Autodesk Inventor part; units mm, degrees
ref_plane "YZ Plane" through (0, 0, 0) normal (1, 0, 0) x (0, 1, 0)
ref_plane "XZ Plane" through (0, 0, 0) normal (0, 1, 0) x (-1, 0, 0)
ref_plane "XY Plane" through (0, 0, 0) normal (0, 0, 1) x (1, 0, 0)
sketch "Sketch1" plane through (0, 0, 0) normal (1, 0, 0) x (0, 1, 0)
  line L0 (0, 0) -> (0, -3.5)
  line L1 (0, -3.5) -> (1.3, -3.5)
  line L2 (1.3, -3.5) -> (1.3, -3.25)
  line L3 (1.3, -3.25) -> (2.3425, -3.25)
  line L4 (2.3425, -3.25) -> (2.3425, -3.5)
  line L5 (2.3425, -3.5) -> (3.6425, -3.5)
  line L6 (3.6425, -3.5) -> (3.6425, -3.25)
  line L7 (3.6425, -3.25) -> (5, -3.25)
  line L8 (5, -3.25) -> (5, 0)
  line L9 (5, 0) -> (0, 0)
  line L10 (5, -2.5) -> (0, -2.5)
  point P0 (1.8212, -3.25)
  dimension "d0" = 3.25
  dimension "d1" = 5
  dimension "d2" = 3.5
  dimension "d3" = 1.3
  dimension "d4" = 1.3
  dimension "d5" = 2.5
revolve "Revolution1" add sketch "Sketch1" angle 360 about axis through (0, 5, 0) along (0, -1, 0) contours L10 L8 L7 L6 L5 L4 L3 L2 L1 L0
equation "\"d4\" = d3"
properties part number "M5 heat set inserts"
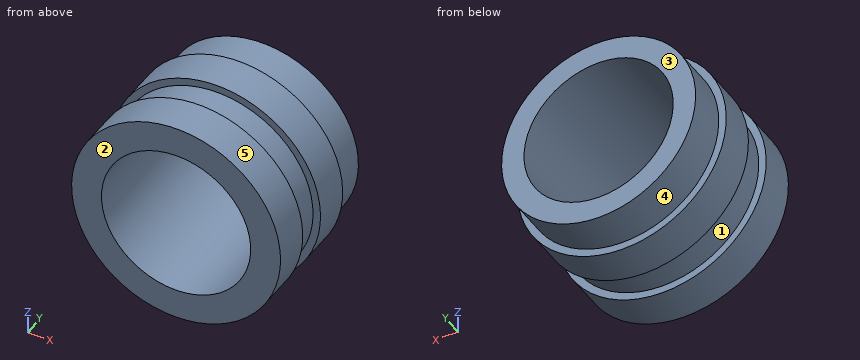
Check sheet for the modelled part. Datum: model origin and axes. Units: mm. Face numbers are marked on the shaded views. A direction names the side the tool comes from. Round coordinates to 2 decimals unless told otherwise and drop trailing zeros. Order: outer loops, then holes, each group sorted by start corner. A loop starts at its lowest first (then second) coordinate and runs counter-clockwise, first axis right, second up.
Q1. Draft check along Y on the marked faces 1, 2 and 3. Enter one of: pulls with the +Y half, pulls with the -Y half, needs draft (parallel to the pull), parting line crosses it, or undercut.
Filled sheet:
face 1: undercut
face 2: pulls with the -Y half
face 3: pulls with the +Y half
Q2. Cross-section at B-B, the plane z = 0. Enter the section's corners in (x, y), plus the area to 3 significant figures.
Filled sheet:
outline: (-3.5, 0) - (-2.5, 0) - (-2.5, 5) - (-3.25, 5) - (-3.25, 3.64) - (-3.5, 3.64) - (-3.5, 2.34) - (-3.25, 2.34) - (-3.25, 1.3) - (-3.5, 1.3) - close; (2.5, 0) - (3.5, 0) - (3.5, 1.3) - (3.25, 1.3) - (3.25, 2.34) - (3.5, 2.34) - (3.5, 3.64) - (3.25, 3.64) - (3.25, 5) - (2.5, 5) - close
area: 8.80 mm2
Q3. Depth check by flat-ended pin: P1, Ø3, axis at x = 2.5, y = 1, coming from the +Z side. Enter the tip coordinate at first touch or a pass-through.
Filled sheet:
P1: stops at z = 3.35
Q4. Set-up check for the marked faces 4 and 5: record each of +Z, -Z, +X, -X, +Y, -Y from which the full face is reachable in a straight line by a thin tool's end or side.
Filled sheet:
face 4: +Y
face 5: +Y, -Y
Q5. Cross-section at A-A, the plane x = 0. Enter the section's corners in (y, z), plus the area to 3 significant figures.
Filled sheet:
outline: (0, -3.5) - (1.3, -3.5) - (1.3, -3.25) - (2.34, -3.25) - (2.34, -3.5) - (3.64, -3.5) - (3.64, -3.25) - (5, -3.25) - (5, -2.5) - (0, -2.5) - close; (0, 2.5) - (5, 2.5) - (5, 3.25) - (3.64, 3.25) - (3.64, 3.5) - (2.34, 3.5) - (2.34, 3.25) - (1.3, 3.25) - (1.3, 3.5) - (0, 3.5) - close
area: 8.80 mm2
Q6. Cross-section at C-C, the plane z = -2.75. Enter the section's corners in (x, y), plus the area to 3 significant figures.
Filled sheet:
outline: (-2.17, 0) - (2.17, 0) - (2.17, 1.3) - (1.73, 1.3) - (1.73, 2.34) - (2.17, 2.34) - (2.17, 3.64) - (1.73, 3.64) - (1.73, 5) - (-1.73, 5) - (-1.73, 3.64) - (-2.17, 3.64) - (-2.17, 2.34) - (-1.73, 2.34) - (-1.73, 1.3) - (-2.17, 1.3) - close
area: 19.6 mm2
Q7. Scan lines: L1, parallel to X at y = 1.8, z = 0; L2, parallel to X at y = 2.45, z = 0; L3, parallel to Z at x = -1.5, y = 1.75. Record each from-to range of solid material in increasing order.
Filled sheet:
L1: x = -3.25 to -2.5, 2.5 to 3.25
L2: x = -3.5 to -2.5, 2.5 to 3.5
L3: z = -2.88 to -2, 2 to 2.88
Q8. Cross-section at D-D, the plane x = -3. Enter the section's corners in (y, z).
Filled sheet:
outline: (0, -1.8) - (1.3, -1.8) - (1.3, -1.25) - (2.34, -1.25) - (2.34, -1.8) - (3.64, -1.8) - (3.64, -1.25) - (5, -1.25) - (5, 1.25) - (3.64, 1.25) - (3.64, 1.8) - (2.34, 1.8) - (2.34, 1.25) - (1.3, 1.25) - (1.3, 1.8) - (0, 1.8) - close
